```python
from build123d import *

# Parameters (mm, degrees)
F0_W      = 122
F0_H      = 57
F1_DEPTH  = 6
F2_R      = 4
F3_R      = 1.5
F3_W      = 8.049835
F3_H      = 2.874941
F4_DEPTH  = 0.5
F5_R      = 6.519395
F6_DEPTH  = 0.5
F7_W      = 88.799998
F7_H      = 42.300004
F8_DEPTH  = 0.1
F9_R      = 3.153566
F9_W      = 2.700009
F9_H      = 13.199998
F10_DEPTH = 0.5


with BuildPart() as f1:
    # F0 (on Top) → F1 (new body)
    with BuildSketch(Plane.XY):
        Rectangle(F0_W, F0_H)
    extrude(amount=F1_DEPTH)

    # F2
    f2_edges = [f1.edges().sort_by_distance(p)[0] for p in [
        (61, 28.5, 3),
        (61, -28.5, 3),
        (-61, 28.5, 3),
        (-61, -28.5, 3),
    ]]
    fillet(f2_edges, radius=F2_R)

    # F3 (on face) → F4 (join)
    with BuildSketch(Plane.XZ.offset(28.5)):
        with Locations((36.866432, 2.725052)):
            Circle(F3_R)
        with Locations((41.46634, 2.725052)):
            Circle(F3_R)
        with Locations((48.941184, 2.725053)):
            Rectangle(F3_W, F3_H)
    extrude(amount=F4_DEPTH)

    # F5 (on face) → F6 (cut)
    with BuildSketch(Plane(origin=(0, 0, 0), x_dir=(1, 0, 0), z_dir=(0, 0, -1))):
        with Locations((-52.800003, 0)):
            Circle(F5_R)
    extrude(amount=-F6_DEPTH, mode=Mode.SUBTRACT)

    # F7 (on face) → F8 (cut)
    with BuildSketch(Plane(origin=(0, 0, 0), x_dir=(1, 0, 0), z_dir=(0, 0, -1))):
        Rectangle(F7_W, F7_H)
    extrude(amount=-F8_DEPTH, mode=Mode.SUBTRACT)

    # F9 (on face) → F10 (cut)
    with BuildSketch(Plane(origin=(0, 0, 0), x_dir=(1, 0, 0), z_dir=(0, 0, -1))):
        with Locations((56.55, 0)):
            Circle(F9_R)
        with Locations((48.599999, 0)):
            Rectangle(F9_W, F9_H)
    extrude(amount=-F10_DEPTH, mode=Mode.SUBTRACT)


solid = f1.part
```
Input: part model. Units: mm. Frame: model coordinates. A direction names the side the tool comes from. Coordinates: 2 decimals unless noted, no trailing zeros. Write each loop counter-clockwise with the first axis right and the second up, starting at its lowest first coordinate (ties: lowest second). Pieces come first, ordered by that corner, then holes. Notation, with made-up numbers: (-27, -9) -> (29, -9) arc R21 ccw to (29, 13) -> close; hole circle Ø8 at (39.5, 51.25). An arc over 180 degrees is marked (long way). Write each question's results on one line, items separated by ' | '.
Item 1: Mould query, pull axis X, two halves, no side actions, for faces 4 (the cylindrical face through (-59.859, 27.297, 3.042)), 5 (the cylindrical face through (-59.313, -0.287, 0.246)), 6 (the flat face through (-1, 0, 0.1)), 7 (the flat face through (49, -29, 3)). Classes: +X half, -X half, draft (parallel to the pull), parting line (faces both ways), or undercut.
Conclusion:
face 4: -X half | face 5: undercut | face 6: undercut | face 7: draft
Item 2: Pin query (flat end, axial travel): pin 1 Ø0.6 at (y, z) = (-28.5, 3) entering from +X; pin 2 Ø1.4 at (x, y) = (49, -1.5) entering from -Z; pin 3 Ø0.6 at (y, z) = (-28.5, 3) entering from -X. Return the tip coordinate at first contact, or that it passes through.
Conclusion:
pin 1: stops at x = 58.52 | pin 2: stops at z = 0.5 | pin 3: stops at x = -58.52
Item 3: Section query B-B on x = -38. Return loops of the section in (y, z), plus the area to 3 significant figures.
Conclusion:
outline: (-28.5, 0) -> (-21.15, 0) -> (-21.15, 0.1) -> (21.15, 0.1) -> (21.15, 0) -> (28.5, 0) -> (28.5, 6) -> (-28.5, 6) -> close | area: 338 mm^2
Item 4: Section query A-A on y = 0. Return loops of the section in (x, z).
Conclusion:
outline: (-61, 0) -> (-59.32, 0) -> (-59.32, 0.5) -> (-46.28, 0.5) -> (-46.28, 0) -> (-44.4, 0) -> (-44.4, 0.1) -> (44.4, 0.1) -> (44.4, 0) -> (47.25, 0) -> (47.25, 0.5) -> (49.95, 0.5) -> (49.95, 0) -> (53.4, 0) -> (53.4, 0.5) -> (59.7, 0.5) -> (59.7, 0) -> (61, 0) -> (61, 6) -> (-61, 6) -> close
Item 5: Material intervals for probe 1 along X at (y, z) = (0, 0.25); probe 2 along Y at (x, z) = (56.55, 0.15); probe 3 along Z at (x, y) = (6, -8.5), sorted ascending.
Conclusion:
probe 1: x = -61 to -59.32, -46.28 to 47.25, 49.95 to 53.4, 59.7 to 61 | probe 2: y = -28.5 to -3.15, 3.15 to 28.5 | probe 3: z = 0.1 to 6
Item 6: Set-up query: faces 1 (the cylindrical face through (59.797, -27.359, 3.042)), 2 (the cylindrical face through (39.968, -28.746, 2.791)), 3 (the flat face through (49, 0, 0.5)). Return all of +Z, -Z, +X, -X, +Y, -Y with unobstructed straight access to the full face (end or side cutting, diameter ignored); none if empty.
Conclusion:
face 1: +Z, -Z, +X, -Y | face 2: -Y | face 3: -Z
